Here's how the part is built. I have some questions about the finished solid (model axes, mm). Round coordinates to 2 decimals unless told otherwise and drop trailing zeros. Order: outer loops, then holes, each group sorted by start corner. A loop starts at its lowest first (then second) coordinate and runs counter-clockwise, first axis right, second up. Notation, with made-up numbers: (33.5, 48) - (42.5, 48) arc R23 ccw to (42.5, 76) - close; hole circle Ø11 at (72, 36.25). An arc over 180 degrees is marked (long way). Answer as a JSON object with one key per item and string values.
```python
from build123d import *

# Parameters (mm, degrees)
SKETCH1_W           = 20
SKETCH1_H           = 20
BOSS_EXTRUDE1_DEPTH = 10
CUT_EXTRUDE1_DEPTH  = 20
CUT_EXTRUDE3_DEPTH  = 20
FILLET1_R           = 0.2


with BuildPart() as part:
    # Sketch1 → Boss-Extrude1 (new body)
    with BuildSketch(Plane(origin=(0, 0, 0), x_dir=(1, 0, 0), z_dir=(0, 1, 0))):
        Rectangle(SKETCH1_W, SKETCH1_H)
    extrude(amount=BOSS_EXTRUDE1_DEPTH)

    # Sketch2 → Cut-Extrude1 (cut)
    with BuildSketch(Plane.XY.offset(10)):
        Polygon((-10, 10), (-10, 0), (0, 10), align=None)
    extrude(amount=-CUT_EXTRUDE1_DEPTH, mode=Mode.SUBTRACT)

    # Sketch3 → Cut-Extrude3 (cut)
    with BuildSketch(Plane.XY.offset(10)):
        Polygon((0, 10), (10, 10), (10, 0), align=None)
    extrude(amount=-CUT_EXTRUDE3_DEPTH, mode=Mode.SUBTRACT)

    # Fillet1
    fillet1_edges = [part.edges().sort_by_distance(p)[0] for p in [
        (0, 10, 0),
    ]]
    fillet(fillet1_edges, radius=FILLET1_R)


solid = part.part
```
1. If I drill on L1, parallel to Y at x = 7.25, z = 2; L2, parallel to Y at x = 4.5, z = -1; L3, parallel to X at y = 1.25, z = 3.75, over which ranges is the centre line in solid material (lowest first)? Write a range as [from, to].
Responses:
{"L1": "[0, 2.75]", "L2": "[0, 5.5]", "L3": "[-8.75, 8.75]"}
2. Imagine slicing it at A-A (y = 7). List the corners of the cut face in (x, z) for me, plus the area to 3 significant figures.
Responses:
{"outline": "(-3, -10) - (3, -10) - (3, 10) - (-3, 10) - close", "area": "120 mm2"}
3. Imagine slicing it at B-B (x = -4.5). List the corners of the cut face in (y, z) for me.
Responses:
{"outline": "(0, -10) - (5.5, -10) - (5.5, 10) - (0, 10) - close"}
4. For P1, Ø10, axis at x = 5.5, z = 7, coming from the +Y side, with a flat end and sliding along its axis, tell me the tip position at first contact or that it passes through.
Responses:
{"P1": "y = 9.5"}
